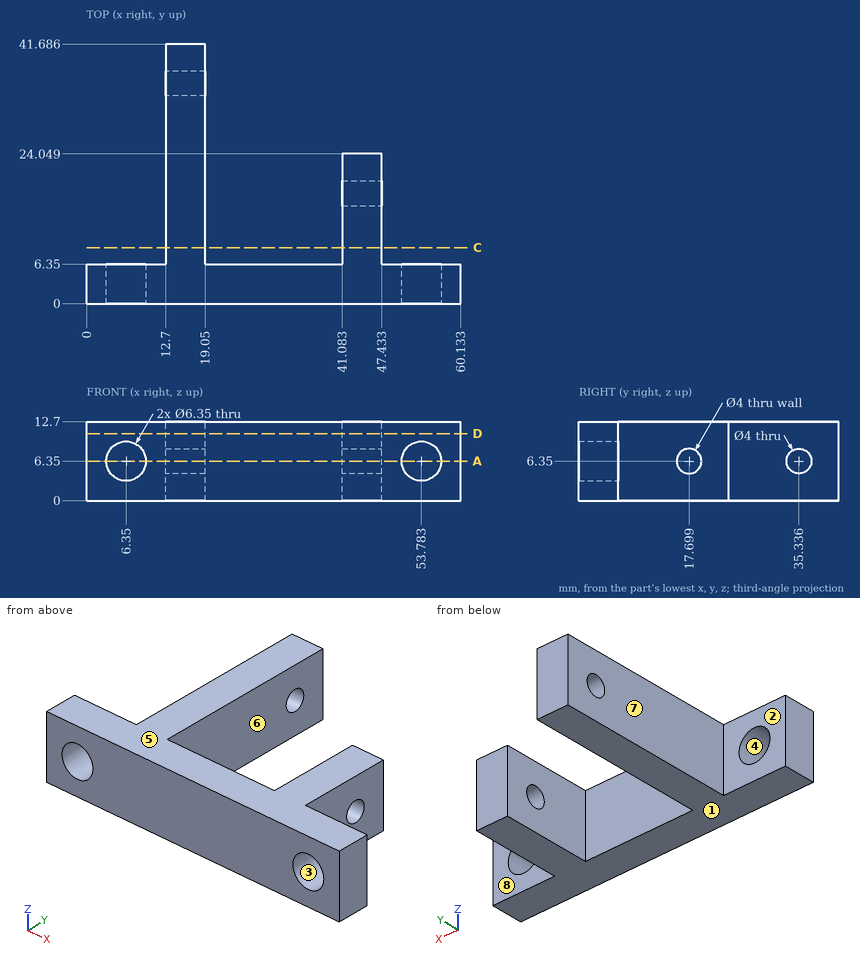
Geometry: see drawing. Coordinates: mm, zero at the bounding-box minimum. A direction names the side the tool comes from. Give positions to 0.01 mm unless a question says otherwise; leave off trailing zeros. Loops run counter-clockwise (first coordinate to the right, second up) from the corner with the lowest first, then second, coordinate; pieces in that order, holes last. Notation, with made-up numbers: (5.5, 35.25) - (49.5, 35.25) arc R7 cw to (49.5, 45.25) - close; hole circle Ø5 at (80, 42). An arc over 180 degrees is marked (long way). Answer as CSV lines item,"result". Start each with the question number.
1. Ray query, L1, parallel to X at y = 23, z = 2; L2, parallel to Z at x = 6.35, y = 2.5 (1 decimal); L3, parallel to Y at x = 43.5, z = 6.35. Return the intervals inside material, ascending.
2. Reachability of the marked faces 4, 5, 6, 7 and 8 from +Z, -Z, +X, -X, +Y, -Y: full face, straight path, thin tool, end or side. Return the list, or none.
3. Draft query along Z for the marked faces 1, 2 and 3. Return one class per face: released by +Z, released by -Z, zero draft, split by the parting line, or undercut.
4. Section D-D, the plane z = 10.75. Return loops of the section in (x, y).
5. Section A-A, the plane z = 6.35. Give the number of separate pieces and of enclosed holes in the cut face, plus the area to 3 significant figures.
6. Section C-C, the plane y = 9. Return loops of the section in (x, z).
7. Pin query (flat end, axial travel): P1, Ø5, axis at x = 43, z = 7, coming from the +Y side; P2, Ø6.5, axis at y = 25, z = 4, coming from the +X side; P3, Ø6.5, axis at x = 7, z = 4, coming from the +Y side; P4, Ø3.5, axis at y = 35.34, z = 6.35, coming from the +X side. Return the tip coordinate at first contact, or that it passes through.
Answers:
1,L1,"x = 12.7 to 19.05, 41.08 to 47.43"
1,L2,"z = 0 to 3.2, 9.5 to 12.7"
1,L3,"y = 0 to 15.7, 19.7 to 24.05"
2,face 4,"+Y, -Y"
2,face 5,"+Z, +X, -X, +Y, -Y"
2,face 6,"+Z, -Z, +Y"
2,face 7,"+Z, -Z, -X, +Y"
2,face 8,"+Z, -Z, +X, +Y"
3,face 1,"released by -Z"
3,face 2,"zero draft"
3,face 3,"undercut"
4,outline,"(0, 0) - (60.13, 0) - (60.13, 6.35) - (47.43, 6.35) - (47.43, 24.05) - (41.08, 24.05) - (41.08, 6.35) - (19.05, 6.35) - (19.05, 41.69) - (12.7, 41.69) - (12.7, 6.35) - (0, 6.35) - close"
5,separate pieces,"5"
5,enclosed holes,"0"
5,area,"587 mm2"
6,outline,"(12.7, 0) - (19.05, 0) - (19.05, 12.7) - (12.7, 12.7) - close; (41.08, 0) - (47.43, 0) - (47.43, 12.7) - (41.08, 12.7) - close"
7,P1,"stops at y = 24.05"
7,P2,"stops at x = 47.43"
7,P3,"stops at y = 6.35"
7,P4,"passes through"
